```python
from build123d import *

# Parameters (mm, degrees)
SKETCH_W        = 25
SKETCH_H        = 45
PAD_DEPTH       = 10
SKETCH001_R     = 11
POCKET_DEPTH    = 7
PAD001_DEPTH    = 3
SKETCH005_W     = 4
SKETCH005_H     = 45.367283
PAD002_DEPTH    = 25
SKETCH003_R     = 6.5
POCKET001_DEPTH = 5
SKETCH007_R     = 2.5
POCKET002_DEPTH = 5


with BuildPart() as part:
    # Sketch → Pad (new body)
    with BuildSketch(Plane.XY):
        with Locations((0, -0.515162)):
            Rectangle(SKETCH_W, SKETCH_H)
    extrude(amount=PAD_DEPTH)

    # Sketch001 (on Face6 of Pad) → Pocket (cut)
    with BuildSketch(Plane.XY.offset(10)):
        with Locations((0, 7.184838)):
            Circle(SKETCH001_R)
    extrude(amount=-POCKET_DEPTH, mode=Mode.SUBTRACT)

    # Sketch004 (on Face3 of Pocket) → Pad001 (join)
    with BuildSketch(Plane.YZ.offset(12.5)):
        Polygon((-23.015162, 0), (21.984838, 0), (-19.015162, -35.367283), (-23.015162, -35.367283), align=None)
    pad001 = extrude(amount=-PAD001_DEPTH)

    # Sketch005 (on Face8 of Pad001) → Pad002 (join)
    with BuildSketch(Plane.YZ.offset(12.5)):
        with Locations((-21.015162, -12.683642)):
            Rectangle(SKETCH005_W, SKETCH005_H)
    extrude(amount=-PAD002_DEPTH)

    # Mirrored: Pad001 across YZ
    add(pad001.mirror(Plane.YZ))

    # Sketch003 (on Face8 of Pocket) → Pocket001 (cut)
    with BuildSketch(Plane.XY.offset(3)):
        with Locations((0, 7.184838)):
            Circle(SKETCH003_R)
    extrude(amount=-POCKET001_DEPTH, mode=Mode.SUBTRACT)

    # Sketch007 (on Face15 of Pocket001) → Pocket002 (cut)
    with BuildSketch(Plane(origin=(0, -19.015162, 0), x_dir=(-1, 0, 0), z_dir=(0, 1, 0))):
        with Locations((0, -6.689823)):
            Circle(SKETCH007_R)
        with Locations((0, -26.003223)):
            Circle(SKETCH007_R)
    extrude(amount=-POCKET002_DEPTH, mode=Mode.SUBTRACT)


solid = part.part
```
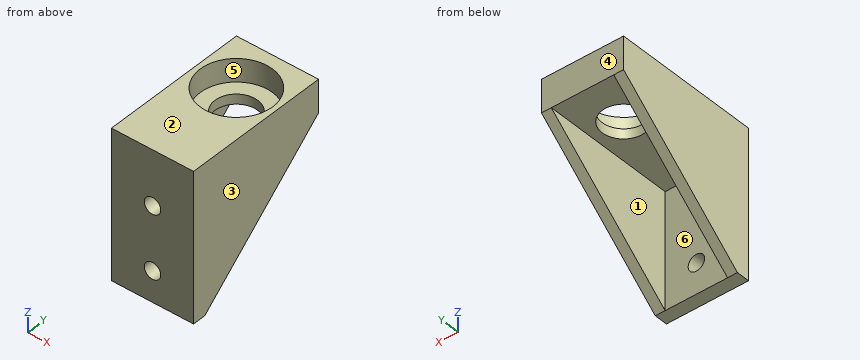
The model under review builds one solid part; all positions refer to its coordinate system, in mm. Face numbers are marked on the shaded views. A direction names the side the tool comes from. Round coordinates to 2 decimals unless told otherwise and drop trailing zeros. Loops run counter-clockwise (first coordinate to the right, second up) from the corner with the lowest first, then second, coordinate; pieces in that order, holes last. Notation, with made-up numbers: M 53.5,82 L 59.5,82 A34 ccw 59.5,114 Z; hole C 26,-12 d6. An arc over 180 degrees is marked long. Write item = value, one per line.
Item 1: The part is to be moulded in two halves that separate along X. For the marked faces 1, 2 and 3, say which applies: released by +X, released by -X, zero draft, split by the parting line, or undercut.
Return value:
face_1 = undercut
face_2 = zero draft
face_3 = released by +X
Item 2: For line 1 (Z direction, x = 0, y = -20.95); line 2 (X direction, y = 7, z = 4); line 3 (Y direction, x = 0, z = 1), list the stretches that pass through material, from the lowest coordinate up. Write a range as [from, to].
Return value:
line_1 = [-35.37, -28.5], [-23.5, -9.19], [-4.19, 10]
line_2 = [-12.5, -11], [11, 12.5]
line_3 = [-23.02, 0.68], [13.68, 21.98]
Item 3: Take a section at D-D on y = -1. Write out the cut boundary in (x, z), then the cut area to 3 significant figures.
Return value:
outline = M -12.5,-19.83 L -9.5,-19.83 L -9.5,0 L 9.5,0 L 9.5,-19.83 L 12.5,-19.83 L 12.5,10 L 7.35,10 L 7.35,3 L -7.35,3 L -7.35,10 L -12.5,10 Z
area = 266 mm2
Item 4: Take a section at C-C on z = -15. Write out the cut boundary in (x, y), then the cut area to 3 significant figures.
Return value:
outline = M -12.5,-23.02 L 12.5,-23.02 L 12.5,4.6 L 9.5,4.6 L 9.5,-19.02 L -9.5,-19.02 L -9.5,4.6 L -12.5,4.6 Z
area = 242 mm2
Item 5: Machinability: for the marked faces 4, 5 and 6, which of the approach directions +Z, -Z, +X, -X, +Y, -Y give a long, thin tool a straight path to every point of the face, cutting with its end or side? Answer none if there is none.
Return value:
face_4 = +Z, -Z, +X, -X, +Y
face_5 = +Z
face_6 = -Z, +Y
Item 6: Insertion check: P1, Ø8, axis at x = -1, z = -14.5, coming from the +Y side; P2, Ø11, axis at x = -4.5, y = 5.5, coming from the +Z side; P3, Ø2, axis at x = 1.5, y = 15.5, coming from the -Z side; P4, Ø10.5, axis at y = 6.5, z = -17, coming from the -X side. Each pin has a flat end and moves straight along its axis. Give the tip position at first contact, or say it passes through.
Return value:
P1 = -19.02
P2 = 3
P3 = 0
P4 = -12.5
Item 7: Take a section at B-B on x = -3.25. Write out the cut boundary in (y, z), then the cut area to 3 significant figures.
Return value:
outline = M -23.02,-35.37 L -19.02,-35.37 L -19.02,0 L 1.56,0 L 1.56,3 L -3.32,3 L -3.32,10 L -23.02,10 Z; M 12.81,0 L 21.98,0 L 21.98,10 L 17.69,10 L 17.69,3 L 12.81,3 Z
area = 411 mm2
Item 8: Take a section at A-A on x = 0. Write out the cut boundary in (y, z), then the cut area to 3 significant figures.
Return value:
outline = M -23.02,-35.37 L -19.02,-35.37 L -19.02,-28.5 L -23.02,-28.5 Z; M -23.02,-23.5 L -19.02,-23.5 L -19.02,-9.19 L -23.02,-9.19 Z; M -23.02,-4.19 L -19.02,-4.19 L -19.02,0 L 0.68,0 L 0.68,3 L -3.82,3 L -3.82,10 L -23.02,10 Z; M 13.68,0 L 21.98,0 L 21.98,10 L 18.18,10 L 18.18,3 L 13.68,3 Z
area = 358 mm2
